Can you work these out from the model? Positions are in its coordinate system, mm. Face numbers are marked on the shaded views. A direction names the side the tool comes from. Give positions to 0.01 mm unless a question says otherwise; leave off trailing zeros. Order: outer loops, then holes, each group sorted by start corner. A loop starts at its lowest first (then second) coordinate and runs counter-clockwise, first axis right, second up.
Item 1: If we mould it in two halves opening along X, with no side actions, what happens to the marked faces 1, 2 and 3? For each: +X half, -X half, draft (parallel to the pull), parting line (faces both ways), or undercut.
Item 2: Which directions (+Z, -Z, +X, -X, +Y, -Y) give clear straight access to the entire face, cutting with the end or side of a thin tool? Please do the marked faces 4 and 5.
Item 3: I want a section at B-B, the plane z = 11.75. Write out the boundary of the cut face in (x, y).
Item 4: I want a section at C-C, the plane x = -5. Write out the boundary of the cut face in (y, z).
Item 5: I'm going to push a flat-ended pin straight in: pin 1 Ø6.5 at (x, z) = (-1, 8) entering from -Y. Where does the tip first touch, or does it pass through?
Item 6: I want a section at A-A, the plane y = 6.5. Write out the boundary of the cut face in (x, z).
Item 7: If I drill on line 1 along X through (y, z) = (6.25, 15.75); line 2 along X through (y, z) = (-4.75, 11.75); line 3 along Y through (x, z) = (-7, 1), over which ranges is the centre line in solid material (lowest first)?
Autodesk Inventor part; units mm, degrees
ref_plane "YZ Plane" through (0, 0, 0) normal (1, 0, 0) x (0, 1, 0)
ref_plane "XZ Plane" through (0, 0, 0) normal (0, 1, 0) x (-1, 0, 0)
ref_plane "XY Plane" through (0, 0, 0) normal (0, 0, 1) x (1, 0, 0)
sketch "Sketch1" plane through (0, 0, 0) normal (0, 0, 1) x (1, 0, 0)
  line L0 (-26.67, 9.906) -> (-8.89, 9.906)
  line L1 (-7.62, 8.636) -> (-7.62, 5.334)
  line L2 (-6.604, 4.318) -> (-6.604, 4.318)
  line L3 (-6.604, 4.318) -> (-6.604, 8.128)
  line L4 (-6.604, 8.128) -> (0, 8.128)
  line L5 (-29.21, 7.366) -> (-29.21, 0)
  line L6 (0, 8.128) -> (0, 0)
  line L7 (0, 0) -> (-29.21, 0)
  arc A0 (-7.62, 5.334) -> (-6.604, 4.318) centre (-6.604, 5.334) ccw
  arc A1 (-7.62, 8.636) -> (-8.89, 9.906) centre (-8.89, 8.636) ccw
  arc A2 (-26.67, 9.906) -> (-29.21, 7.366) centre (-26.67, 7.366) ccw
  line L8 (26.67, 9.906) -> (8.89, 9.906)
  line L9 (7.62, 8.636) -> (7.62, 5.334)
  line L10 (6.604, 4.318) -> (6.604, 4.318)
  line L11 (6.604, 4.318) -> (6.604, 8.128)
  line L12 (6.604, 8.128) -> (0, 8.128)
  line L13 (29.21, 7.366) -> (29.21, 0)
  line L14 (0, 0) -> (29.21, 0)
  arc A3 (6.604, 4.318) -> (7.62, 5.334) centre (6.604, 5.334) ccw
  arc A4 (8.89, 9.906) -> (7.62, 8.636) centre (8.89, 8.636) ccw
  arc A5 (29.21, 7.366) -> (26.67, 9.906) centre (26.67, 7.366) ccw
  line L15 (-26.67, -9.906) -> (-8.89, -9.906)
  line L16 (-7.62, -8.636) -> (-7.62, -8.128)
  line L17 (-6.604, -4.318) -> (-6.604, -8.128)
  line L18 (-6.604, -8.128) -> (0, -8.128)
  line L19 (-29.21, -7.366) -> (-29.21, 0)
  line L20 (0, -8.128) -> (0, 0)
  arc A6 (-8.89, -9.906) -> (-7.62, -8.636) centre (-8.89, -8.636) ccw
  arc A7 (-29.21, -7.366) -> (-26.67, -9.906) centre (-26.67, -7.366) ccw
  line L21 (29.21, -7.366) -> (29.21, 0)
  arc A8 (26.67, -9.906) -> (29.21, -7.366) centre (26.67, -7.366) ccw
  line L22 (26.67, -9.906) -> (8.89, -9.906)
  arc A9 (7.62, -8.636) -> (8.89, -9.906) centre (8.89, -8.636) ccw
  line L23 (6.604, -4.318) -> (6.604, -8.128)
  line L24 (6.604, -8.128) -> (0, -8.128)
  line L25 (-7.62, -8.636) -> (-7.62, -5.334)
  line L26 (-7.62, -5.334) -> (-7.62, -5.334)
  line L27 (-6.604, -4.318) -> (-6.604, -4.318)
  arc A10 (-6.604, -4.318) -> (-7.62, -5.334) centre (-6.604, -5.334) ccw
  line L28 (7.62, -8.636) -> (7.62, -5.334)
  line L29 (7.62, -5.334) -> (7.62, -5.334)
  line L30 (6.604, -4.318) -> (6.604, -4.318)
  arc A11 (7.62, -5.334) -> (6.604, -4.318) centre (6.604, -5.334) ccw
  point P0 (-7.62, -4.318)
  dimension "d0" = 29.21
  dimension "d1" = 7.62
  dimension "d2" = 1.016
  dimension "d3" = 5.588
  dimension "d4" = 9.906
  dimension "d5" = 8.128
  dimension "d6" = 1.016
  dimension "d7" = 1.27
  dimension "d8" = 2.54
  dimension "d9" = 1.016
  dimension "d10" = 1.016
extrude "Extrusion1" add sketch "Sketch1" along normal blind 22.86
properties part number "ARTHURw5.5bAutomobloxConnectorPiece"
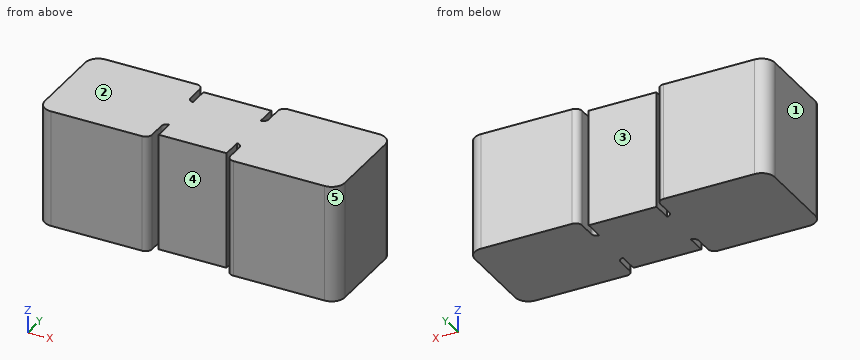
Results list:
1. face 1: -X half
1. face 2: draft
1. face 3: undercut
2. face 4: +Z, -Z, -Y
2. face 5: +Z, -Z, +X, -Y
3. outline: (-29.21, -7.37) arc R2.54 ccw to (-26.67, -9.91) - (-8.89, -9.91) arc R1.27 ccw to (-7.62, -8.64) - (-7.62, -5.33) arc R1.02 cw to (-6.6, -4.32) - (-6.6, -8.13) - (6.6, -8.13) - (6.6, -4.32) arc R1.02 cw to (7.62, -5.33) - (7.62, -8.64) arc R1.27 ccw to (8.89, -9.91) - (26.67, -9.91) arc R2.54 ccw to (29.21, -7.37) - (29.21, 7.37) arc R2.54 ccw to (26.67, 9.91) - (8.89, 9.91) arc R1.27 ccw to (7.62, 8.64) - (7.62, 5.33) arc R1.02 cw to (6.6, 4.32) - (6.6, 8.13) - (-6.6, 8.13) - (-6.6, 4.32) arc R1.02 cw to (-7.62, 5.33) - (-7.62, 8.64) arc R1.27 ccw to (-8.89, 9.91) - (-26.67, 9.91) arc R2.54 ccw to (-29.21, 7.37) - close
4. outline: (-8.13, 0) - (8.13, 0) - (8.13, 22.86) - (-8.13, 22.86) - close
5. pin 1: stops at y = -8.13
6. outline: (-29.21, 0) - (-7.62, 0) - (-7.62, 22.86) - (-29.21, 22.86) - close; (-6.6, 0) - (6.6, 0) - (6.6, 22.86) - (-6.6, 22.86) - close; (7.62, 0) - (29.21, 0) - (29.21, 22.86) - (7.62, 22.86) - close
7. line 1: x = -29.21 to -7.62, -6.6 to 6.6, 7.62 to 29.21
7. line 2: x = -29.21 to -7.44, -6.6 to 6.6, 7.44 to 29.21
7. line 3: y = -4.4 to 4.4
